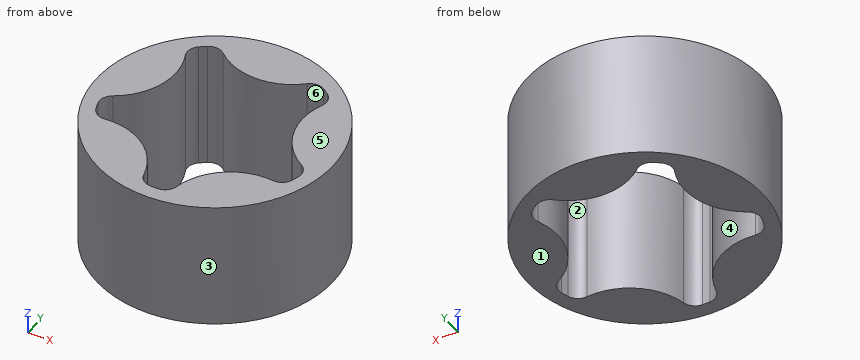
from build123d import *

# Parameters (mm, degrees)
SKETCH1_R          = 20.2565
BASE_EXTRUDE_DEPTH = 21.971


with BuildPart() as part:
    # Sketch1 → Base-Extrude (new body)
    with BuildSketch(Plane.XY):
        Circle(SKETCH1_R)
        with BuildLine():
            ThreePointArc((-9.962871848, 14.803096865), (-10.488146149, 14.435694739), (-10.999885021, 14.049662693))
            ThreePointArc((-10.999885021, 14.049662693), (-11.807615401, 12.807242878), (-11.683709562, 11.330529398))
            ThreePointArc((-11.683709562, 11.330529398), (-11.301861211, 3.672197312), (-16.112237674, -2.299078665))
            ThreePointArc((-16.112237674, -2.299078665), (-17.080470009, -3.420934942), (-17.157278449, -4.900845691))
            ThreePointArc((-17.157278449, -4.900845691), (-16.970176949, -5.513944739), (-16.761174663, -6.11992779))
            ThreePointArc((-16.761174663, -6.11992779), (-15.829165617, -7.272053868), (-14.386438629, -7.610541975))
            ThreePointArc((-14.386438629, -7.610541975), (-6.984934365, -9.613937375), (-2.792401513, -16.034103011))
            ThreePointArc((-2.792401513, -16.034103011), (-2.024653036, -17.301619337), (-0.640909388, -17.831986076))
            ThreePointArc((-0.640909388, -17.831986076), (0, -17.8435), (0.640909388, -17.831986076))
            ThreePointArc((0.640909388, -17.831986076), (2.024653036, -17.301619337), (2.792401513, -16.034103011))
            ThreePointArc((2.792401513, -16.034103011), (6.984934365, -9.613937375), (14.386438629, -7.610541975))
            ThreePointArc((14.386438629, -7.610541975), (15.829165617, -7.272053868), (16.761174663, -6.11992779))
            ThreePointArc((16.761174663, -6.11992779), (16.970176949, -5.513944739), (17.157278449, -4.900845691))
            ThreePointArc((17.157278449, -4.900845691), (17.080470009, -3.420934942), (16.112237674, -2.299078665))
            ThreePointArc((16.112237674, -2.299078665), (11.301861211, 3.672197312), (11.683709562, 11.330529398))
            ThreePointArc((11.683709562, 11.330529398), (11.807615401, 12.807242878), (10.999885021, 14.049662693))
            ThreePointArc((10.999885021, 14.049662693), (10.488146149, 14.435694739), (9.962871848, 14.803096865))
            ThreePointArc((9.962871848, 14.803096865), (8.531657973, 15.187365269), (7.165509005, 14.613194253))
            ThreePointArc((7.165509005, 14.613194253), (0, 11.883480127), (-7.165509005, 14.613194253))
            ThreePointArc((-7.165509005, 14.613194253), (-8.531657973, 15.187365269), (-9.962871848, 14.803096865))
        make_face(mode=Mode.SUBTRACT)
    extrude(amount=BASE_EXTRUDE_DEPTH)


solid = part.part
Geometry: final body of the model. Coordinates: model frame, mm. Face numbers are marked on the shaded views. A direction names the side the tool comes from. Give positions to 0.01 mm unless a question says otherwise; leave off trailing zeros. Write each loop counter-clockwise with the first axis right and the second up, starting at its lowest first coordinate (ties: lowest second). Pieces come first, ordered by that corner, then holes.
(1) Cut plane C-C, the plane y = 0. Return loops of the section in (x, z).
(2) Mould query, pull axis X, two halves, no side actions, for the marked faces 3, 4, 5 and 6. Classes: released by +X, released by -X, zero draft, split by the parting line, or undercut.
(3) Ray query, line 1 (Y direction, x = 7, z = 11.75); line 2 (Y direction, x = -0.5, z = 6); line 3 (X direction, y = -17, z = 5.75). Return the intervals inside material, ascending.
(4) Cut plane B-B, the plane z = 4. Return loops of the section in (x, y).
(5) Access query for the marked faces 1 and 2. Directions: +Z, -Z, +X, -X, +Y, -Y. A direction counts if a zero-diameter tool reaches every point of the face in a straight line with its end or side. Return the directions, or none.
(6) Cut plane A-A, the plane x = 0. Return loops of the section in (y, z).
(7) First-contact query: P1, Ø1.5, axis at x = -2.5, z = 5.5, coming from the -Y side; P2, Ø8, axis at y = -10.5, z = 7, coming from the -X side; P3, Ø2, axis at x = 11, z = 9, coming from the -Y side; P4, Ø12, axis at x = 8.5, y = -6.5, coming from the -Z side. Flat tips, straight axial feed; report the tip coordinate or a pass-through.
Values follow:
1. outline: (-20.26, 0) - (-13.36, 0) - (-13.36, 21.97) - (-20.26, 21.97) - close; (13.36, 0) - (20.26, 0) - (20.26, 21.97) - (13.36, 21.97) - close
2. face 3: split by the parting line
2. face 4: undercut
2. face 5: zero draft
2. face 6: undercut
3. line 1: y = -19.01 to -9.6, 14.47 to 19.01
3. line 2: y = -20.25 to -17.84, 11.9 to 20.25
3. line 3: x = -11.01 to -2.32, 2.32 to 11.01
4. outline: circle Ø40.51 at (0, 0); hole (-17.16, -4.9) arc R17.84 ccw to (-16.76, -6.12) arc R2.29 ccw to (-14.39, -7.61) arc R10.77 cw to (-2.79, -16.03) arc R2.29 ccw to (-0.64, -17.83) arc R17.84 ccw to (0.64, -17.83) arc R2.29 ccw to (2.79, -16.03) arc R10.77 cw to (14.39, -7.61) arc R2.29 ccw to (16.76, -6.12) arc R17.84 ccw to (17.16, -4.9) arc R2.29 ccw to (16.11, -2.3) arc R10.77 cw to (11.68, 11.33) arc R2.29 ccw to (11, 14.05) arc R17.84 ccw to (9.96, 14.8) arc R2.29 ccw to (7.17, 14.61) arc R10.77 cw to (-7.17, 14.61) arc R2.29 ccw to (-9.96, 14.8) arc R17.84 ccw to (-11, 14.05) arc R2.29 ccw to (-11.68, 11.33) arc R10.77 cw to (-16.11, -2.3) arc R2.29 ccw to start
5. face 1: -Z, +X, -X, +Y, -Y
5. face 2: +Z, -Z
6. outline: (-20.26, 0) - (-17.84, 0) - (-17.84, 21.97) - (-20.26, 21.97) - close; (11.88, 0) - (20.26, 0) - (20.26, 21.97) - (11.88, 21.97) - close
7. P1: stops at y = -20.18
7. P2: stops at x = -19.19
7. P3: stops at y = -17.62
7. P4: stops at z = 0
